```python
from build123d import *

# Parameters (mm, degrees)
F0_R          = 5.75
F0_R_2        = 4.75
F1_DEPTH      = 100
F2_R          = 4.75
F2_R_2        = 3.5
F3_DEPTH      = 10
F3_DEPTH_BACK = 10


with BuildPart() as f1:
    # F0 (on Top) → F1 (new body)
    with BuildSketch(Plane.XY):
        Circle(F0_R)
        Circle(F0_R_2, mode=Mode.SUBTRACT)
    extrude(amount=-F1_DEPTH)

    # F2 (on face) → F3 (join, two sides)
    with BuildSketch(Plane.XY) as f3_sk:
        Circle(F2_R)
        Circle(F2_R_2, mode=Mode.SUBTRACT)
    extrude(amount=F3_DEPTH)
    extrude(f3_sk.sketch, amount=-F3_DEPTH_BACK)


solid = f1.part
```
Check sheet for the modelled part. Datum: model origin and axes. Units: mm. A direction names the side the tool comes from. Round coordinates to 2 decimals unless told otherwise and drop trailing zeros. Loops run counter-clockwise (first coordinate to the right, second up) from the corner with the lowest first, then second, coordinate; pieces in that order, holes last. Notation, with made-up numbers: (28, -11.5) - (35, -11.5) arc R19 cw to (35, -5.5) - close; hole circle Ø8 at (-11, 54). An arc over 180 degrees is marked (long way). Answer as a JSON object with one key per item and string values. Group by question number.
Q1. Sectioned sample at C-C, the plane z = -21. Enter the section's corners in (x, y).
Q2. Scan lines: line 1 along Y through (x, z) = (0, 6.5); line 2 along Y through (x, z) = (0, -36); line 3 along X through (y, z) = (-0.25, -31.5). Record each from-to range of solid material in increasing order. Write a range as [from, to].
Q3. Sectioned sample at A-A, the plane y = 0. Enter the section's corners in (x, z), plus the area to 3 significant figures.
Q4. Set-up check for faces 1 (the face through (2.192, -4.214, 4.93)), 2 (the face through (1, 5, -100)), 3 (the face through (-4, 0, -10)): record each of +Z, -Z, +X, -X, +Y, -Y from which the full face is reachable in a straight line by a thin tool's end or side.
Q5. Gauge pin test, flat ends, axial feed: P1, Ø4, axis at y = -1.5, z = -15.5, coming from the -X side; P2, Ø1, axis at x = -2.5, z = -3, coming from the -Y side; P3, Ø1, axis at x = 2.5, z = -4, coming from the +Y side; P4, Ø5, axis at x = 0.5, y = -1.5, coming from the -Z side. Record the tip position at first contact, or that the pin passes through.
Q6. Mould release check, pull along Y, two halves, no side actions. Record for faces 4 (the face through (-0.75, 5.7, -49.3)), 5 (the face through (2.192, -4.214, -54.37)), 6 (the face through (1, 5, 0)): released by +Y, released by -Y, zero draft, split by the parting line, or undercut.
Solution:
{
 "1": {"outline": "circle Ø11.5 at (0, 0); hole circle Ø9.5 at (0, 0)"},
 "2": {"line 1": "y = [-4.75, -3.5], [3.5, 4.75]", "line 2": "y = [-5.75, -4.75], [4.75, 5.75]", "line 3": "x = [-5.74, -4.74], [4.74, 5.74]"},
 "3": {"outline": "(-5.75, -100) - (-4.75, -100) - (-4.75, -10) - (-3.5, -10) - (-3.5, 10) - (-4.75, 10) - (-4.75, 0) - (-5.75, 0) - close; (3.5, -10) - (4.75, -10) - (4.75, -100) - (5.75, -100) - (5.75, 0) - (4.75, 0) - (4.75, 10) - (3.5, 10) - close", "area": "250 mm²"},
 "4": {"face 1": "+Z", "face 2": "-Z, +X, -X, +Y, -Y", "face 3": "-Z"},
 "5": {"P1": "stops at x = -5.75", "P2": "stops at y = -5.39", "P3": "stops at y = 5.39", "P4": "stops at z = -10"},
 "6": {"face 4": "split by the parting line", "face 5": "undercut", "face 6": "zero draft"}
}
